from build123d import *

# Parameters (mm, degrees)
SM_BASE_FLANGE_1_DEPTH   = 436
CUT_EXTRUDE_1_DEPTH      = 10
CUT_EXTRUDE_1_DEPTH_BACK = 10
SKETCH_2_W               = 12.842994449
SKETCH_2_H               = 79.921875175
SKETCH_2_W_2             = 14.142108975
SKETCH_2_H_2             = 88.32377597


# Sheet-metal steps are written as plain solids
with BuildPart() as part:
    # Sketch 1 → 基体-法兰1 (new body)
    with BuildSketch(Plane.XY):
        with BuildLine():
            Line((-10, 0), (-2.7366, 0))
            ThreePointArc((-2.7366, 0), (-0.801531583, 0.801531583), (0, 2.7366))
            Line((0, 2.7366), (0, 19.2634))
            ThreePointArc((0, 19.2634), (0.215745145, 19.784254855), (0.7366, 20))
            Line((0.7366, 20), (29.2634, 20))
            ThreePointArc((29.2634, 20), (29.784254855, 19.784254855), (30, 19.2634))
            Line((30, 19.2634), (30, 2.7366))
            ThreePointArc((30, 2.7366), (30.801531583, 0.801531583), (32.7366, 0))
            Line((32.7366, 0), (40, 0))
            Line((40, 0), (40, 2))
            Line((40, 2), (32.7366, 2))
            ThreePointArc((32.7366, 2), (32.215745145, 2.215745145), (32, 2.7366))
            Line((32, 2.7366), (32, 19.2634))
            ThreePointArc((32, 19.2634), (31.198468417, 21.198468417), (29.2634, 22))
            Line((29.2634, 22), (0.7366, 22))
            ThreePointArc((0.7366, 22), (-1.198468417, 21.198468417), (-2, 19.2634))
            Line((-2, 19.2634), (-2, 2.7366))
            ThreePointArc((-2, 2.7366), (-2.215745145, 2.215745145), (-2.7366, 2))
            Line((-2.7366, 2), (-10, 2))
            Line((-10, 2), (-10, 0))
        make_face()
    extrude(amount=SM_BASE_FLANGE_1_DEPTH)

    # Sketch 2 → 切除-拉伸1 (cut, two sides: drawn at the far end of the back side and taken through both)
    with BuildSketch(Plane(origin=(0, 2, 0), x_dir=(1, 0, 0), z_dir=(0, 1, 0)).offset(-CUT_EXTRUDE_1_DEPTH_BACK)):
        with Locations((-8.421497225, -36.039062413)):
            Rectangle(SKETCH_2_W, SKETCH_2_H)
        with Locations((-9.071054487, -404.161887985)):
            Rectangle(SKETCH_2_W_2, SKETCH_2_H_2)
    extrude(amount=CUT_EXTRUDE_1_DEPTH + CUT_EXTRUDE_1_DEPTH_BACK, mode=Mode.SUBTRACT)


solid = part.part
CAD build for the part. Positions are in the model's coordinates, mm. A direction names the side the tool comes from. Give positions to 0.01 mm unless a question says otherwise; leave off trailing zeros. Loops run counter-clockwise (first coordinate to the right, second up) from the corner with the lowest first, then second, coordinate; pieces in that order, holes last. Notation, with made-up numbers: M -10,15.25 L 33,15.25 A20 cw 33,26.25 Z; hole C 37,-34 d6. An arc over 180 degrees is marked long. Answer in a Markdown table with one row per item. Add a question column.
Item 1: Band-saw the part on C-C on x = 20. Give the cut face in (y, z).
Item 2: Mould opens along X. For faces 1 (the face through (30, 11, 215)), 2 (the face through (32, 11, 215)), 3 (the face through (-6, 2, 216)) say: +X half, -X half, draft (parallel to the pull), parting line (faces both ways), or undercut.
Item 3: Probe probe 1 along X at (y, z) = (4, 409); probe 2 along Y at (x, z) = (38, 416.5); probe 3 along Y at (x, z) = (2, 30). List the from-to ranges inside material, lowest first.
Item 4: Drop flat-ended pins along their axis: P1, Ø13, axis at y = 12, z = 118, coming from the +X side; P2, Ø8, axis at x = 37, z = 256, coming from the +Y side; P3, Ø3, axis at x = -6.5, y = 1, coming from the +Z side; P4, Ø2, axis at x = 1.5, y = 16.5, coming from the -Z side. Give the stop position or say it passes through.
Item 5: Band-saw the part on A-A on y = 10.5. Give the cut face in (x, z), then the cut area to 3 significant figures.
Item 6: Band-saw the part on B-B on z = 342. Give the cut face in (x, y).
Item 7: Band-saw the part on D-D on z = 32.5. Give the cut face in (x, y).
Item 8: Tool access for faces 4 (the face through (15, 20, 215)), 5 (the face through (16, 21, 0)), 6 (the face through (36, 2, 215)): list every direction of +Z, -Z, +X, -X, +Y, -Y with a clear straight run to the whole face (end or side of a thin tool).
Reply:
| question | item | result |
|---|---|---|
| 1 | outline | M 20,0 L 22,0 L 22,436 L 20,436 Z |
| 2 | face 1 | undercut |
| 2 | face 2 | +X half |
| 2 | face 3 | draft |
| 3 | probe 1 | x = -2 to 0, 30 to 32 |
| 3 | probe 2 | y = 0 to 2 |
| 3 | probe 3 | y = 20 to 22 |
| 4 | P1 | stops at x = 32 |
| 4 | P2 | stops at y = 2 |
| 4 | P3 | stops at z = 360 |
| 4 | P4 | passes through |
| 5 | outline | M -2,0 L 0,0 L 0,436 L -2,436 Z; M 30,0 L 32,0 L 32,436 L 30,436 Z |
| 5 | area | 1,740 mm^2 |
| 6 | outline | M -10,0 L -2.74,0 A2.74 ccw 0,2.74 L 0,19.26 A0.74 cw 0.74,20 L 29.26,20 A0.74 cw 30,19.26 L 30,2.74 A2.74 ccw 32.74,0 L 40,0 L 40,2 L 32.74,2 A0.74 cw 32,2.74 L 32,19.26 A2.74 ccw 29.26,22 L 0.74,22 A2.74 ccw -2,19.26 L -2,2.74 A0.74 cw -2.74,2 L -10,2 Z |
| 7 | outline | M -2,0.1 A2.74 ccw 0,2.74 L 0,19.26 A0.74 cw 0.74,20 L 29.26,20 A0.74 cw 30,19.26 L 30,2.74 A2.74 ccw 32.74,0 L 40,0 L 40,2 L 32.74,2 A0.74 cw 32,2.74 L 32,19.26 A2.74 ccw 29.26,22 L 0.74,22 A2.74 ccw -2,19.26 Z |
| 8 | face 4 | +Z, -Z, -Y |
| 8 | face 5 | -Z, +X, -X, +Y, -Y |
| 8 | face 6 | +Z, -Z, +X, +Y |
